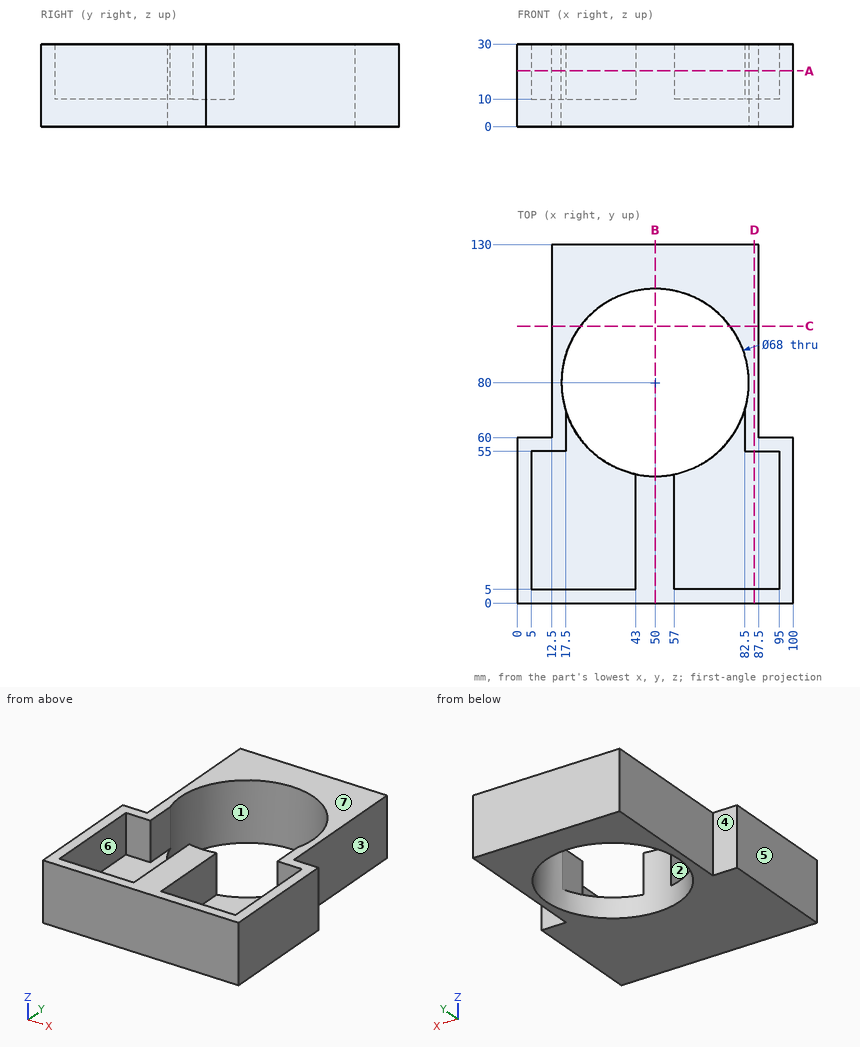
The drawing under review shows one solid part. Ordinate dimensions are in mm from its lowest x, y, z. A direction names the side the tool comes from. Give positions to 0.01 mm unless a question says otherwise; leave off trailing zeros. Write each loop counter-clockwise with the first axis right and the second up, starting at its lowest first coordinate (ties: lowest second). Pieces come first, ordered by that corner, then holes. Notation, with made-up numbers: (-33.5, 78.5) -> (23.5, 78.5) arc R22 ccw to (23.5, 115.5) -> close; hole circle Ø7 at (23.5, -12.75). An arc over 180 degrees is marked (long way). Answer in a Markdown table with one row per item.
(1) For the marked faces 1, 2, 3 and 4, list the 3-axis set-ups (+Z, -Z, +X, -X, +Y, -Y) from which the entire face can be reached by the end or side of a thin tool; tool diameter is ignored.
Results:
| item | result |
|---|---|
| face 1 | +Z, -Z |
| face 2 | +Z |
| face 3 | +Z, -Z, +X, +Y |
| face 4 | +Z, -Z, -X, +Y |
(2) Clearance check with flat-ended pins moving along their axes: pin 1 (7.5 mm diameter, centred on y = 65, z = 21, fed in from -X); pin 2 (6 mm diameter, centred on y = 103.5, z = 9, fed in from +X); pin 3 (4 mm diameter, centred on x = 97, z = 11.5, fed in from +Y). State where each tip first meets the part, or that it passes through.
Results:
| item | result |
|---|---|
| pin 1 | x = 12.5 |
| pin 2 | x = 87.5 |
| pin 3 | y = 60 |
(3) Consider section C-C (y = 100.5). State the section outline as (x, z) points.
Results:
| item | result |
|---|---|
| outline | (12.5, 0) -> (22.88, 0) -> (22.88, 30) -> (12.5, 30) -> close; (77.12, 0) -> (87.5, 0) -> (87.5, 30) -> (77.12, 30) -> close |
(4) To check wall thickness, follow probe 1 along X at (y, z) = (29.5, 16.5); probe 2 along X at (y, z) = (80.5, 18.75); probe 3 along Y at (x, z) = (50, 6.5). State the ranges of each line that lie inside material, in increasing order.
Results:
| item | result |
|---|---|
| probe 1 | 0 to 5, 43 to 57, 95 to 100 |
| probe 2 | 12.5 to 16, 84 to 87.5 |
| probe 3 | 0 to 46, 114 to 130 |
(5) Consider section A-A (z = 20.25). State the section outline as (x, y) points.
Results:
| item | result |
|---|---|
| outline | (0, 0) -> (100, 0) -> (100, 60) -> (87.5, 60) -> (87.5, 130) -> (12.5, 130) -> (12.5, 60) -> (0, 60) -> close; hole (5, 5) -> (43, 5) -> (43, 46.73) arc R34 ccw to (57, 46.73) -> (57, 5) -> (95, 5) -> (95, 55) -> (82.5, 55) -> (82.5, 70.01) arc R34 ccw (long way) to (17.5, 70.01) -> (17.5, 55) -> (5, 55) -> close |
(6) Consider section D-D (x = 86). State the section outline as (y, z) points.
Results:
| item | result |
|---|---|
| outline | (0, 0) -> (130, 0) -> (130, 30) -> (55, 30) -> (55, 10) -> (5, 10) -> (5, 30) -> (0, 30) -> close |
(7) Mouldability with a two-part tool opening along X and no side actions: class the marked faces 5, 6 and 7 as +X half, -X half, draft (parallel to the pull), parting line (faces both ways), or undercut.
Results:
| item | result |
|---|---|
| face 5 | -X half |
| face 6 | undercut |
| face 7 | draft |
(8) Consider section B-B (x = 50). State the section outline as (y, z) points, then the cut area to 3 significant figures.
Results:
| item | result |
|---|---|
| outline | (0, 0) -> (46, 0) -> (46, 30) -> (0, 30) -> close; (114, 0) -> (130, 0) -> (130, 30) -> (114, 30) -> close |
| area | 1,860 mm2 |
